For this review, take the finished solid that the model builds, in its own axes (mm). A direction names the side the tool comes from. Coordinates: 2 decimals unless noted, no trailing zeros. Loops run counter-clockwise (first coordinate to the right, second up) from the corner with the lowest first, then second, coordinate; pieces in that order, holes last.
1. Clearance check with flat-ended pins moving along their axes: P1, Ø1, axis at y = 2.5, z = 11.5, coming from the -X side; P2, Ø1.5, axis at y = 9.5, z = 17.5, coming from the -X side; P3, Ø6, axis at x = 0, z = 10, coming from the -Y side; P4, Ø8, axis at x = 8, y = 5, coming from the +Z side. State where each tip first meets the part, or that it passes through.
2. Take a section at B-B, the plane x = 0. State the section outline as (y, z) points.
3. To check wall thickness, follow probe 1 along Z at (x, y) = (0, 3.5); probe 2 along Z at (x, y) = (9.75, 2.5); probe 3 along X at (y, z) = (0, 20.25). State the ranges of each line that lie inside material, in increasing order.
4. Mouldability with a two-part tool opening along Z and no side actions: class faces 4 (the face through (1.075, 2.732, 21.686)), 5 (the face through (0, 0, 0)), 6 (the face through (3, -10, 14)), 7 (the face through (3, -3, 16)) as pulls with the +Z half, pulls with the -Z half, needs draft (parallel to the pull), parting line crosses it, or undercut.
5. Take a section at C-C, the plane y = 0. State the section outline as (x, z) points, then the cut area to 3 significant figures.
6. Machinability: for faces 1 (the face through (0.867, -3.905, 19.944)), 2 (the face through (-0.325, -0.14, 8.536)), 3 (the face through (-2.17, 9.76, 7.92)), which of the approach directions +Z, -Z, +X, -X, +Y, -Y give a long, thin tool a straight path to every point of the face, cutting with its end or side? Answer none if there is none.
7. Take a section at A-A, the plane y = -12. State the section outline as (x, z) points.
8. Take a section at D-D, the plane x = -12.75. State the section outline as (y, z) points.
Autodesk Fusion 360 part; units mm, degrees
sketch "Sketch1" plane through (0, 0, 0) normal (0, 0, 1) x (1, 0, 0)
  circle A0 centre (0, 0) radius 15
  dimension "d1" = 30
extrude "Extrude1" add sketch "Sketch1" along normal blind 16
ref_plane "WorkPlane2" through (0, 0, 2) normal (0, 0, 1) x (1, 0, 0)
sketch "Sketch2" plane through (0, 0, 2) normal (0, 0, 1) x (1, 0, 0)
  circle A0 centre (0, 0) radius 10
  circle A1 centre (0, 0) radius 15
  dimension "d6" = 20
extrude "Extrude2" cut sketch "Sketch2" along normal blind 12
sketch "Sketch3" plane through (0, 0, 16) normal (0, 0, 1) x (-1, 0, 0)
  circle A0 centre (0, 0) radius 15
  circle A1 centre (0, 0) radius 4
  dimension "d9" = 8
extrude "Extrude3" add sketch "Sketch3" along normal blind 8 contours A1
sketch "Sketch4" plane through (0, 0, 0) normal (0, 1, 0) x (1, 0, 0)
  circle A0 centre (0, -20) radius 2
  circle A1 centre (0, -10) radius 1.5
  dimension "d12" = 4
  dimension "d13" = 3
extrude "Extrude4" cut sketch "Sketch4" along normal blind 5 contours A0
extrude "Extrude5" cut sketch "Sketch4" along normal mid plane 40 contours A1
sketch "Sketch5" plane through (0, 0, 24) normal (0, 0, 1) x (-1, 0, 0)
  circle A0 centre (0, 0) radius 4
  circle A1 centre (0, 0) radius 2.5
  dimension "d18" = 5
extrude "Extrude6" cut sketch "Sketch5" against normal blind 10 contours A1
Results list:
1. P1: stops at x = -9.8
1. P2: passes through
1. P3: stops at y = -10
1. P4: stops at z = 16
2. outline: (-15, 0) - (15, 0) - (15, 2) - (10, 2) - (10, 8.5) - (-10, 8.5) - (-10, 2) - (-15, 2) - close; (-15, 14) - (-10, 14) - (-10, 11.5) - (10, 11.5) - (10, 14) - (15, 14) - (15, 16) - (4, 16) - (4, 18) - (2.5, 18) - (2.5, 14) - (-2.5, 14) - (-2.5, 24) - (-4, 24) - (-4, 16) - (-15, 16) - close; (2.5, 22) - (4, 22) - (4, 24) - (2.5, 24) - close
3. probe 1: z = 0 to 8.5, 11.5 to 18, 22 to 24
3. probe 2: z = 0 to 2, 14 to 16
3. probe 3: x = -4 to -2.5, 2.5 to 4
4. face 4: undercut
4. face 5: pulls with the -Z half
4. face 6: undercut
4. face 7: pulls with the +Z half
5. outline: (-15, 0) - (15, 0) - (15, 2) - (10, 2) - (10, 14) - (15, 14) - (15, 16) - (4, 16) - (4, 24) - (2.5, 24) - (2.5, 14) - (-2.5, 14) - (-2.5, 24) - (-4, 24) - (-4, 16) - (-15, 16) - (-15, 14) - (-10, 14) - (-10, 2) - (-15, 2) - close; hole circle Ø3 at (0, 10)
5. area: 367 mm2
6. face 1: +Z
6. face 2: +Y, -Y
6. face 3: none
7. outline: (-9, 0) - (9, 0) - (9, 2) - (-9, 2) - close; (-9, 14) - (9, 14) - (9, 16) - (-9, 16) - close
8. outline: (-7.9, 0) - (7.9, 0) - (7.9, 2) - (-7.9, 2) - close; (-7.9, 14) - (7.9, 14) - (7.9, 16) - (-7.9, 16) - close
